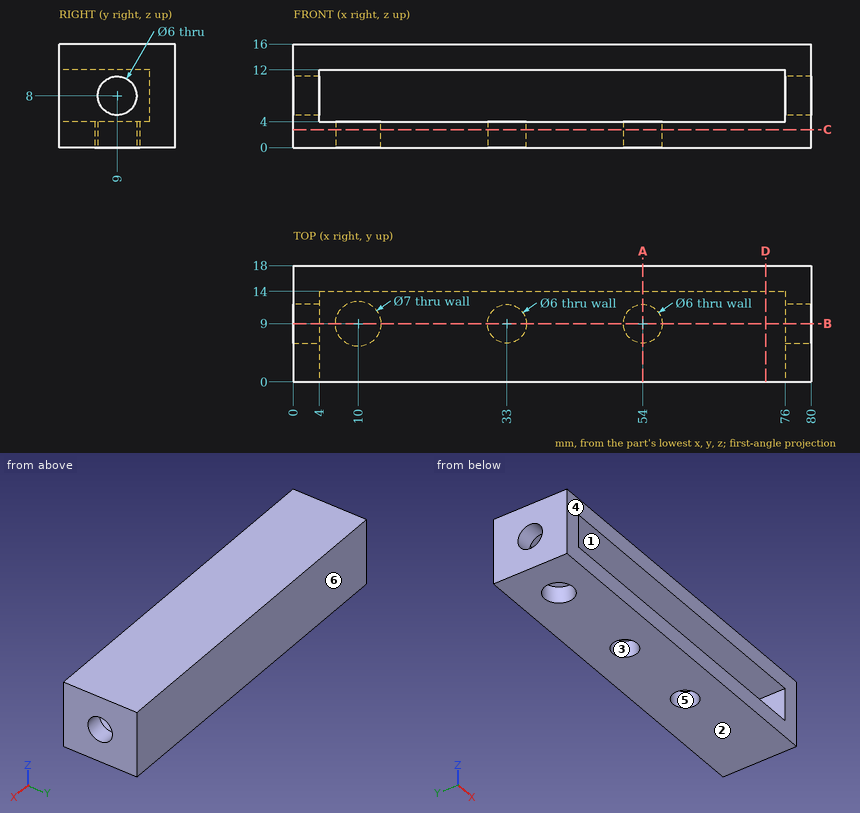
Study the drawing (mm; zero at the part's minimum x, y, z) and answer. A direction names the side the tool comes from. Round coordinates to 2 decimals unless told otherwise and drop trailing zeros. Write each loop counter-clockwise with the first axis right and the second up, starting at its lowest first coordinate (ties: lowest second). Pieces come first, ordered by that corner, then holes. Notation, with made-up numbers: (53, 15.5) - (59, 15.5) arc R21 ccw to (59, 35.5) - close; hole circle Ø7 at (37.25, 18.25). An arc over 180 degrees is marked (long way). Use a Markdown table: item, result. Add a question column.
1. Flat-ended cylindrical pins translate along their axes: P1, Ø7, axis at y = 9, z = 8, coming from the +X side; P2, Ø6.5, axis at x = 45.5, z = 7.5, coming from the -Y side; P3, Ø5.5, axis at x = 33, y = 9, coming from the -Z side. Find the tip coordinate at first contact, or state that the pin passes through.
2. The part is cut by section A-A (x = 54). Write down the section's boundary in (y, z), and give its area (3 significant figures).
3. For a pull along Y with two mould halves and no side action, classify the marked faces 4, 5 and 6 as +Y half, -Y half, draft (parallel to the pull), parting line (faces both ways), or undercut.
4. The part is cut by section D-D (x = 73). Write down the section's boundary in (y, z).
5. Consider line 1 (Z direction, x = 56, y = 3.25); line 2 (Y direction, x = 10, z = 2.75); line 3 (X direction, y = 4.25, z = 11.5). Determine where each line is inside the solid, lowest interval first.
6. A tool of negligible diameter and unlimited length cuts with its end or side. For the marked faces 1, 2 and 3, from which of +Z, -Z, +X, -X, +Y, -Y can it reach the whole face along a straight path? Write none if from no direction.
7. The part is cut by section B-B (y = 9). Write down the section's boundary in (x, z).
8. The part is cut by section C-C (z = 2.75). Write down the section's boundary in (x, y).
Reported:
| question | item | result |
|---|---|---|
| 1 | P1 | x = 80 |
| 1 | P2 | y = 14 |
| 1 | P3 | z = 12 |
| 2 | outline | (0, 0) - (6, 0) - (6, 4) - (0, 4) - close; (0, 12) - (14, 12) - (14, 4) - (12, 4) - (12, 0) - (18, 0) - (18, 16) - (0, 16) - close |
| 2 | area | 152 mm^2 |
| 3 | face 4 | -Y half |
| 3 | face 5 | undercut |
| 3 | face 6 | +Y half |
| 4 | outline | (0, 0) - (18, 0) - (18, 16) - (0, 16) - (0, 12) - (14, 12) - (14, 4) - (0, 4) - close |
| 5 | line 1 | 0 to 4, 12 to 16 |
| 5 | line 2 | 0 to 5.5, 12.5 to 18 |
| 5 | line 3 | 0 to 4, 76 to 80 |
| 6 | face 1 | -Y |
| 6 | face 2 | -Z, +X, -X, +Y, -Y |
| 6 | face 3 | -Z |
| 7 | outline | (0, 0) - (6.5, 0) - (6.5, 4) - (4, 4) - (4, 5) - (0, 5) - close; (0, 11) - (4, 11) - (4, 12) - (76, 12) - (76, 11) - (80, 11) - (80, 16) - (0, 16) - close; (13.5, 0) - (30, 0) - (30, 4) - (13.5, 4) - close; (36, 0) - (51, 0) - (51, 4) - (36, 4) - close; (57, 0) - (80, 0) - (80, 5) - (76, 5) - (76, 4) - (57, 4) - close |
| 8 | outline | (0, 0) - (80, 0) - (80, 18) - (0, 18) - close; hole circle Ø7 at (10, 9); hole circle Ø6 at (33, 9); hole circle Ø6 at (54, 9) |
